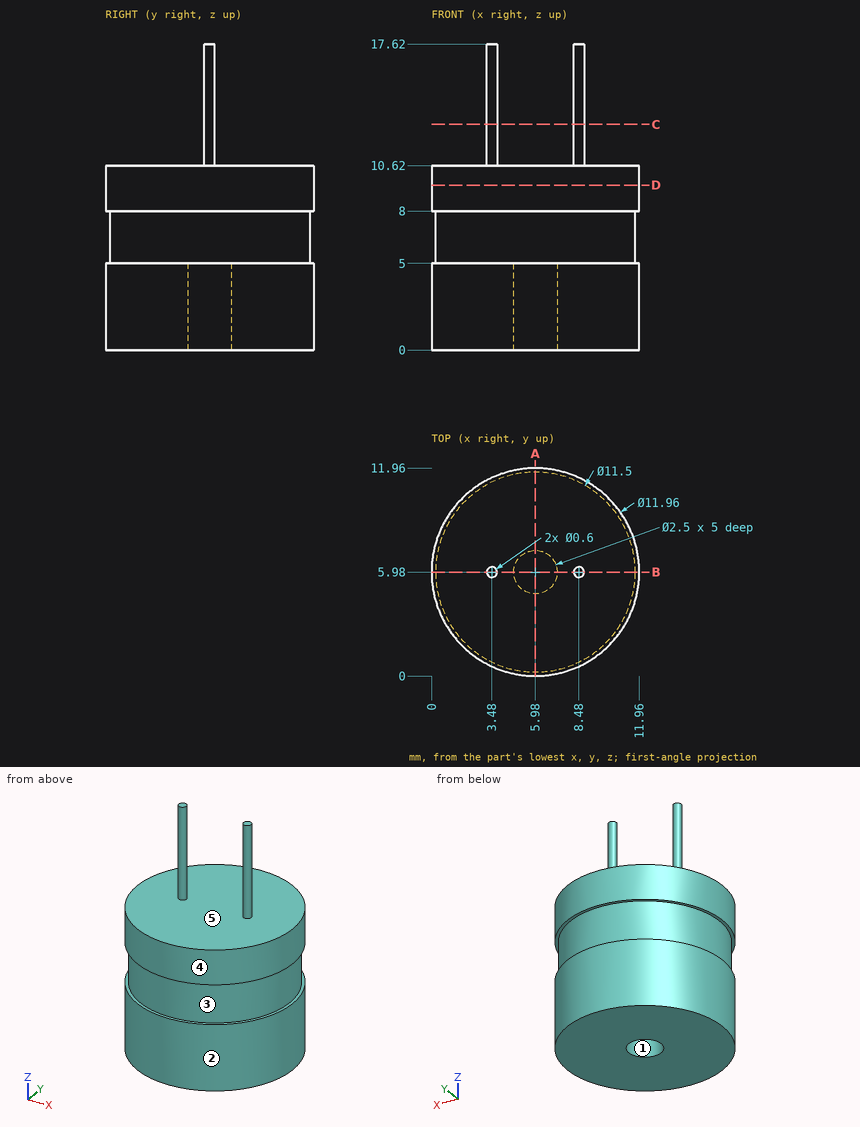
Answer from the drawing. Dimensions are ordinates in mm from the lowest x, y and z of the part. A direction names the side the tool comes from. Give positions to 0.01 mm unless a question says otherwise; leave off trailing zeros. Write each loop counter-clockwise with the first axis right and the second up, starting at its lowest first coordinate (ties: lowest second). Pieces come first, ordered by that corner, then holes. Notation, with made-up numbers: (-1, 0.5) - (37, 0.5) arc R29 cw to (37, 39.5) - close; hole circle Ø2 at (69, 32). An arc over 180 degrees is marked (long way). One line per item, written item: value. Start each with the question number.
1. Find section A-A (x = 5.98). Write down the section's boundary in (y, z).
2. For a pull along Z with two mould halves and no side action, classify the marked faces 3, 4 and 5 as +Z half, -Z half, draft (parallel to the pull), parting line (faces both ways), or undercut.
3. Find section B-B (y = 5.98). Write down the section's boundary in (x, z).
4. For the marked faces 1 and 2, determine the directions among +Z, -Z, +X, -X, +Y, -Y from which every point of the face is accessible in a straight line to the end or side of a thin tool.
5. Consider probe 1 along Y at (x, z) = (5.98, 3.5); probe 2 along Z at (x, y) = (10.75, 6); probe 3 along X at (y, z) = (6.5, 3.5). Determine where each line is inside the solid, lowest interval first.
6. Given pin 1 (1.5 mm diameter, centred on x = 3.5, z = 11, fed in from +Y); pin 2 (1 mm diameter, centred on x = 3.5, y = 2.5, fed in from +Z); pin 3 (1 mm diameter, centred on y = 6.5, z = 15.5, fed in from -X), each flat-ended and moving along its own axis, determine where each tip first touches the part or whether it passes through.
7. Find section D-D (z = 9.5). Write down the section's boundary in (x, y), then the cut area to 3 significant figures.
8. Find section C-C (z = 13). Write down the section's boundary in (x, y).
Geometry results:
1. outline: (0, 0) - (4.73, 0) - (4.73, 5) - (7.23, 5) - (7.23, 0) - (11.96, 0) - (11.96, 5) - (11.73, 5) - (11.73, 8) - (11.96, 8) - (11.96, 10.62) - (0, 10.62) - (0, 8) - (0.23, 8) - (0.23, 5) - (0, 5) - close
2. face 3: undercut
2. face 4: draft
2. face 5: +Z half
3. outline: (0, 0) - (4.73, 0) - (4.73, 5) - (7.23, 5) - (7.23, 0) - (11.96, 0) - (11.96, 5) - (11.73, 5) - (11.73, 8) - (11.96, 8) - (11.96, 10.62) - (8.78, 10.62) - (8.78, 17.62) - (8.18, 17.62) - (8.18, 10.62) - (3.78, 10.62) - (3.78, 17.62) - (3.18, 17.62) - (3.18, 10.62) - (0, 10.62) - (0, 8) - (0.23, 8) - (0.23, 5) - (0, 5) - close
4. face 1: -Z
4. face 2: +Z, -Z
5. probe 1: 0 to 4.73, 7.23 to 11.96
5. probe 2: 0 to 10.62
5. probe 3: 0.02 to 4.84, 7.12 to 11.94
6. pin 1: y = 11.67
6. pin 2: z = 10.62
6. pin 3: x = 3.18
7. outline: circle Ø11.96 at (5.98, 5.98)
7. area: 112 mm2
8. outline: circle Ø0.6 at (3.48, 5.98); circle Ø0.6 at (8.48, 5.98)
